Design review of the part built by this model. Coordinates are the model's own, in mm. A direction names the side the tool comes from. Round coordinates to 2 decimals unless told otherwise and drop trailing zeros. Order: outer loops, then holes, each group sorted by start corner. A loop starts at its lowest first (then second) coordinate and runs counter-clockwise, first axis right, second up.
from build123d import *

# Parameters (mm, degrees)
F2_DEPTH = 152.4
F3_DEPTH = 101.6


with BuildPart() as f2:
    # F0 (on Top) → F2 (new body)
    with BuildSketch(Plane.XY):
        Polygon((63.179306, 63.188269), (-63.818872, 63.868547), (-63.818872, -63.811731), (63.179306, -63.811731), align=None)
    extrude(amount=F2_DEPTH)

    # F1 (on face) → F3 (cut)
    with BuildSketch(Plane.XY):
        Polygon((-13.281766, 63.979113), (-64.081766, 63.979113), (-64.081766, 13.179113), align=None)
    extrude(amount=F3_DEPTH, mode=Mode.SUBTRACT)


solid = f2.part
1) Take a section at B-B on x = -38.5. Give the boundary of the cut face in (y, z).
Results:
outline: (-63.81, 0) - (38.76, 0) - (38.76, 101.6) - (63.73, 101.6) - (63.73, 152.4) - (-63.81, 152.4) - close
2) For faces 1 (the face through (-1, 1, 0)), 2 (the face through (-39.09, 38.17, 50.09)), list the 3-axis set-ups (+Z, -Z, +X, -X, +Y, -Y) from which the entire face can be reached by the end or side of a thin tool; tool diameter is ignored.
Results:
face 1: -Z, +X, -X, +Y, -Y
face 2: -Z, -X, +Y
3) Take a section at A-A on z = 42. Give the boundary of the cut face in (x, y).
Results:
outline: (-63.82, -63.81) - (63.18, -63.81) - (63.18, 63.19) - (-13.66, 63.6) - (-63.82, 13.44) - close
4) Take a section at C-C on y = 30. Give the boundary of the cut face in (x, z).
Results:
outline: (-63.82, 101.6) - (-47.26, 101.6) - (-47.26, 0) - (63.18, 0) - (63.18, 152.4) - (-63.82, 152.4) - close
5) Clearance check with flat-ended pins moving along their axes: P1, Ø6, axis at x = -50, y = -27, coming from the -Z side; P2, Ø12, axis at x = -22, z = 65.5, coming from the +Y side; P3, Ø10, axis at x = 45, z = 35.5, coming from the +Y side; P4, Ø1, axis at x = 32, z = 134.5, coming from the +Y side. State where each tip first meets the part, or that it passes through.
Results:
P1: stops at z = 0
P2: stops at y = 61.26
P3: stops at y = 63.31
P4: stops at y = 63.36
6) To check wall thickness, follow line 1 along Y through (x, z) = (-17, 105); line 2 along Z through (x, y) = (-44, 37); line 3 along Y through (x, z) = (54.5, 26.5). State the ranges of each line that lie inside material, in increasing order.
Results:
line 1: y = -63.81 to 63.62
line 2: z = 101.6 to 152.4
line 3: y = -63.81 to 63.23
